from build123d import *

# Parameters (mm, degrees)
F1_DEPTH = 20
F2_R     = 2.25
F3_DEPTH = 21.501
F5_R     = 4
F6_DEPTH = 14.501


with BuildPart() as f1:
    # F0 (on Front) → F1 (new body)
    with BuildSketch(Plane.XZ):
        with BuildLine():
            ThreePointArc((-12.961481, 1), (0, 13), (12.961481, 1))
            Line((12.961481, 1), (22.477767, 1))
            ThreePointArc((22.477767, 1), (0, 22.5), (-22.477767, 1))
            Line((-22.477767, 1), (-12.961481, 1))
        make_face()
    extrude(amount=F1_DEPTH)

    # F2 (on face) → F3 (cut, through all)
    with BuildSketch(Plane(origin=(0, 0, 1), x_dir=(1, 0, 0), z_dir=(0, 0, -1))):
        with Locations((-17.25, 10)):
            Circle(F2_R)
        with Locations((17.25, 10)):
            Circle(F2_R)
    extrude(amount=-F3_DEPTH, mode=Mode.SUBTRACT)

    # F5 (on offset) → F6 (cut, through all)
    with BuildSketch(Plane.XY.offset(8)):
        with Locations((-17.25, -10)):
            Circle(F5_R)
        with Locations((17.25, -10)):
            Circle(F5_R)
    extrude(amount=F6_DEPTH, mode=Mode.SUBTRACT)


solid = f1.part
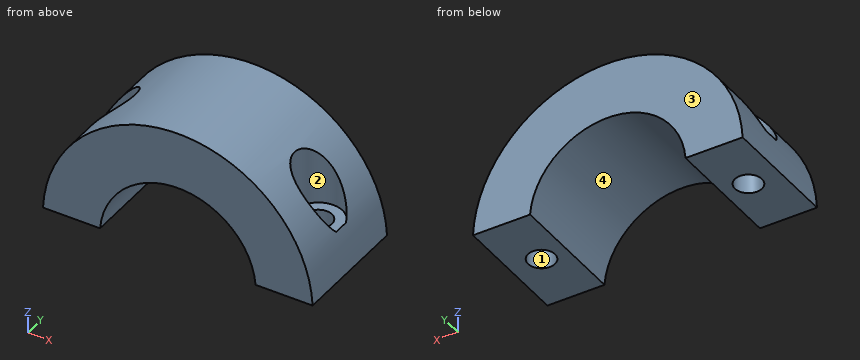
Check sheet for the modelled part. Datum: model origin and axes. Units: mm. Face numbers are marked on the shaded views. Give positions to 0.01 mm unless a question says otherwise; leave off trailing zeros. Loops run counter-clockwise (first coordinate to the right, second up) from the corner with the lowest first, then second, coordinate; pieces in that order, holes last. Notation, with made-up numbers: M 28.25,87.25 L 63.25,87.25 A28 cw 63.25,105.25 Z; hole C -9,10.5 d7. An arc over 180 degrees is marked long. Return JSON: item names as keys, results as strings. Group by question number.
1. Cross-section at B-B on x = 17.25. Record the boundary of the cut face in (y, z), plus the area to 3 significant figures.
2. Mould release check, pull along Y, two halves, no side actions. Record for the marked faces 1, 2, 3 and 4: released by +Y, released by -Y, zero draft, split by the parting line, or undercut.
3. Cross-section at A-A on y = -10. Record the boundary of the cut face in (x, z).
4. Cross-section at C-C on z = 11.75. Record the boundary of the cut face in (x, y), plus the area to 3 significant figures.
5. Go/stop test with flat-tipped pins: pin 1 (3 mm diameter, centred on x = 8, y = -12, fed in from +Z); pin 2 (5 mm diameter, centred on x = -17, y = -10.5, fed in from +Z); pin 3 (4 mm diameter, centred on y = -4, z = 13.5, fed in from +X). Record where each tip stops, or that it passes through.
6. Cross-section at D-D on z = 15.75. Record the boundary of the cut face in (x, y).
7. Thickness scan on L1, parallel to Y at x = -17, z = 10.25; L2, parallel to X at y = -10, z = 2.5; L3, parallel to X at y = -11.5, z = 3.25. Record the ranges inside material, lowest first.
Return value:
{
 "1": {"outline": "M -20,1 L -12.25,1 L -12.25,8 L -14,8 L -14,14.45 L -20,14.45 Z; M -7.75,1 L 0,1 L 0,14.45 L -6,14.45 L -6,8 L -7.75,8 Z", "area": "186 mm^2"},
 "2": {"face 1": "undercut", "face 2": "undercut", "face 3": "released by +Y", "face 4": "zero draft"},
 "3": {"outline": "M -22.48,1 L -19.5,1 L -19.5,8 L -21.03,8 A22.5 ccw Z; M -15,1 L -12.96,1 A13 cw 12.96,1 L 15,1 L 15,8 L 13.25,8 L 13.25,18.18 A22.5 ccw -13.25,18.18 L -13.25,8 L -15,8 Z; M 19.5,1 L 22.48,1 A22.5 ccw 21.03,8 L 19.5,8 Z"},
 "4": {"outline": "M -19.19,-20 L -5.56,-20 L -5.56,0 L -19.19,0 L -19.19,-6.5 A4 cw long -19.19,-13.5 Z; M 5.56,-20 L 19.19,-20 L 19.19,-13.5 A4 cw long 19.19,-6.5 L 19.19,0 L 5.56,0 Z", "area": "465 mm^2"},
 "5": {"pin 1": "z = 21.54", "pin 2": "z = 8", "pin 3": "x = 19.34"},
 "6": {"outline": "M -16.07,-20 L 16.07,-20 L 16.07,-13.82 A4 cw 16.07,-6.18 L 16.07,0 L -16.07,0 L -16.07,-6.18 A4 cw -16.07,-13.82 Z"},
 "7": {"L1": "-20 to -13.99, -6.01 to 0", "L2": "-22.36 to -19.5, -15 to -12.76, 12.76 to 15, 19.5 to 22.36", "L3": "-22.26 to -18.93, -15.57 to -12.59, 12.59 to 15.57, 18.93 to 22.26"}
}
